Answer from the drawing. Dimensions are ordinates in mm from the lowest x, y and z of the part. A direction names the side the tool comes from. Round coordinates to 2 decimals unless told otherwise and drop trailing zeros. Write each loop counter-clockwise with the first axis right and the second up, starting at its lowest first coordinate (ties: lowest second). Pieces come first, ordered by that corner, then holes. Notation, with made-up numbers: (-2, 77.5) - (47, 77.5) arc R25 cw to (47, 113.5) - close; hole circle Ø2 at (65, -26.5). An arc over 180 degrees is marked (long way). Answer as a JSON object with one key per item and string values.
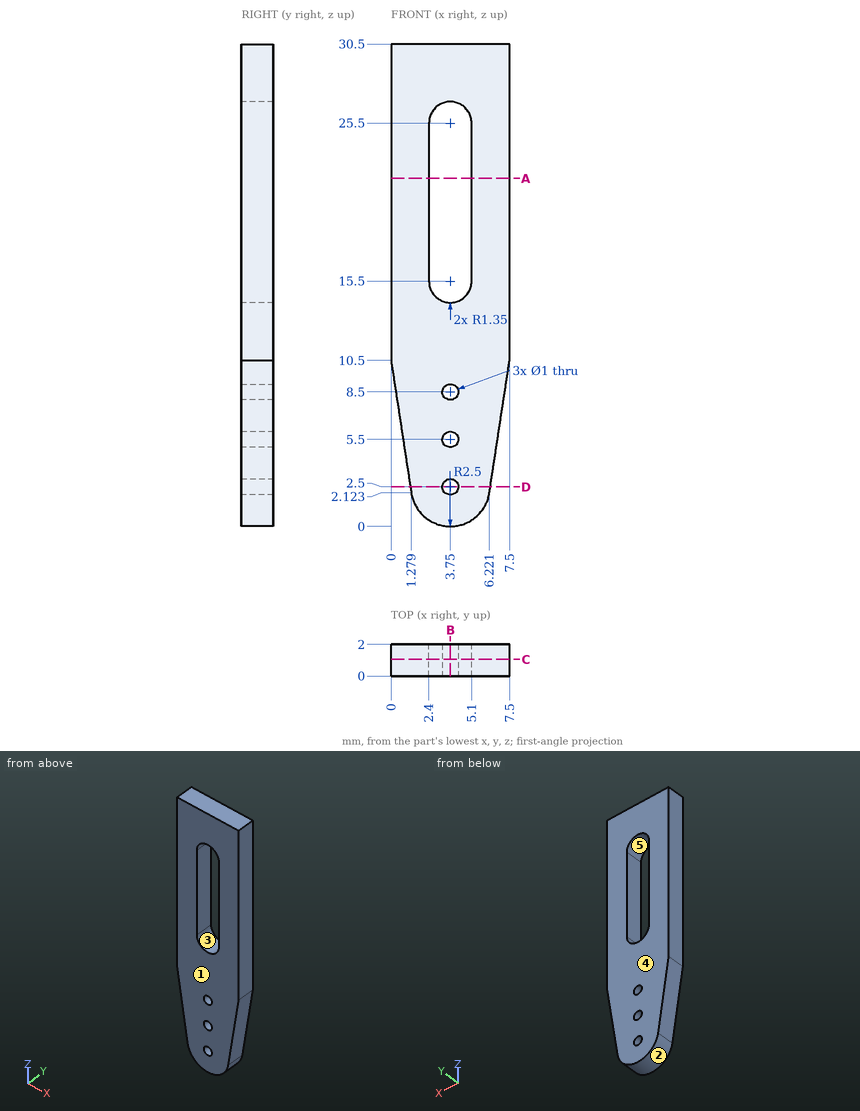
Item 1: Determine the mould class of the marked faces 1, 2 and 3 for opening direction Z: pulls with the +Z half, pulls with the -Z half, needs draft (parallel to the pull), parting line crosses it, or undercut.
Results found:
{"face 1": "needs draft", "face 2": "pulls with the -Z half", "face 3": "undercut"}
Item 2: A cutting plane is placed at A-A (z = 22). Write down the section's boundary in (x, y).
Results found:
{"outline": "(0, 0) - (2.4, 0) - (2.4, 2) - (0, 2) - close; (5.1, 0) - (7.5, 0) - (7.5, 2) - (5.1, 2) - close"}
Item 3: A cutting plane is placed at D-D (z = 2.5). Write down the section's boundary in (x, y).
Results found:
{"outline": "(1.22, 0) - (3.25, 0) - (3.25, 2) - (1.22, 2) - close; (4.25, 0) - (6.28, 0) - (6.28, 2) - (4.25, 2) - close"}
Item 4: A cutting plane is placed at B-B (x = 3.75). Write down the section's boundary in (y, z), and give its area (3 significant figures).
Results found:
{"outline": "(0, 0) - (2, 0) - (2, 2) - (0, 2) - close; (0, 3) - (2, 3) - (2, 5) - (0, 5) - close; (0, 6) - (2, 6) - (2, 8) - (0, 8) - close; (0, 9) - (2, 9) - (2, 14.15) - (0, 14.15) - close; (0, 26.85) - (2, 26.85) - (2, 30.5) - (0, 30.5) - close", "area": "29.6 mm²"}
Item 5: For the marked faces 4 and 5, determine the directions among +Z, -Z, +X, -X, +Y, -Y from which every point of the face is accessible in a straight line to the end or side of a thin tool.
Results found:
{"face 4": "+Z, -Z, +X, -X, +Y", "face 5": "+Y, -Y"}
Item 6: Consider line 1 along X through (y, z) = (1.15, 15.5); line 2 along Z through (x, y) = (3.5, 1) (1 decimal); line 3 along X through (y, z) = (0.45, 5.5). Determine where each line is inside the solid, lowest interval first.
Results found:
{"line 1": "0 to 2.4, 5.1 to 7.5", "line 2": "0 to 2.1, 2.9 to 5.1, 5.9 to 8.1, 8.9 to 14.2, 26.8 to 30.5", "line 3": "0.76 to 3.25, 4.25 to 6.74"}
Item 7: A cutting plane is placed at C-C (y = 1.05). Write down the section's boundary in (x, z).
Results found:
{"outline": "(0, 10.5) - (1.28, 2.12) arc R2.5 ccw to (6.22, 2.12) - (7.5, 10.5) - (7.5, 30.5) - (0, 30.5) - close; hole (2.4, 15.5) arc R1.35 ccw to (5.1, 15.5) - (5.1, 25.5) arc R1.35 ccw to (2.4, 25.5) - close; hole circle Ø1 at (3.75, 2.5); hole circle Ø1 at (3.75, 5.5); hole circle Ø1 at (3.75, 8.5)"}
